Geometry: final body of the model. Coordinates: model frame, mm. Face numbers are marked on the shaded views. A direction names the side the tool comes from. Give positions to 0.01 mm unless a question says otherwise; leave off trailing zeros. Loops run counter-clockwise (first coordinate to the right, second up) from the corner with the lowest first, then second, coordinate; pieces in that order, holes last.
1. Section D-D, the plane x = 13.5. Output: boundary loops of the cut face in (y, z) (3 decimals), then the cut area to 3 significant figures.
2. First-contact query: P1, Ø8, axis at x = 0, y = -22.5, coming from the -Z side; P2, Ø1.6, axis at y = 2.5, z = 1, coming from the -X side; P3, Ø3, axis at x = -17, y = 14.5, coming from the +Z side; P4, Ø14, axis at x = -4.5, y = 25, coming from the +Z side (3 decimals). Flat tips, straight axial feed; report the tip coordinate or a pass-through.
3. Section C-C, the plane z = 43.5. Output: boundary loops of the cut face in (x, y), then the cut area to 3 significant figures.
4. Section B-B, the plane x = -10. Output: boundary loops of the cut face in (y, z) (3 decimals), then the cut area to 3 significant figures.
5. Material intervals for line 1 along Z through (x, y) = (-7.5, -28.5) (3 decimals); line 2 along Z through (x, y) = (-10, 11.5) (3 decimals); line 3 along X through (y, z) = (-14, 2.5), sorted ascending.
6. Access query for the marked faces 1, 2, 3 and 4. Directions: +Z, -Z, +X, -X, +Y, -Y. A direction counts if a zero-diameter tool reaches every point of the face in a straight line with its end or side. Return the directions, or none.
7. Section A-A, the plane y = -13.5. Output: boundary loops of the cut face in (x, z) (3 decimals), then the cut area to 3 significant figures.
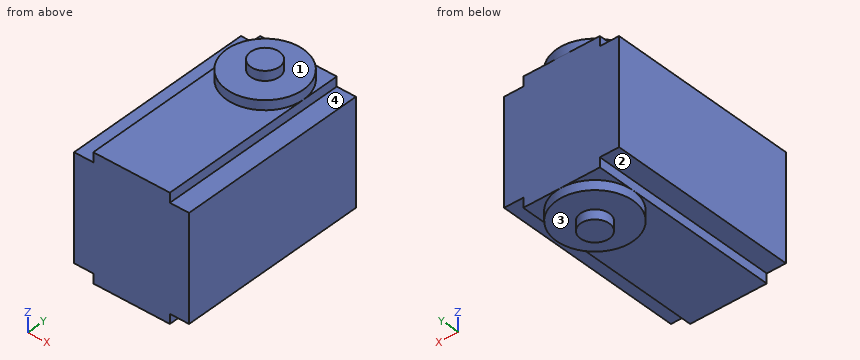
from build123d import *

# Parameters (mm, degrees)
SKETCH1_W           = 38.1
SKETCH1_H           = 63.5
BOSS_EXTRUDE1_DEPTH = 41.275
SKETCH2_R           = 12.7
BOSS_EXTRUDE2_DEPTH = 3.175
SKETCH3_R           = 4.7625
BOSS_EXTRUDE3_DEPTH = 3.175
SKETCH5_W           = 6.35
SKETCH5_H           = 63.5
CUT_EXTRUDE1_DEPTH  = 3.175


with BuildPart() as part:
    # Sketch1 → Boss-Extrude1 (new body)
    with BuildSketch(Plane.XY):
        Rectangle(SKETCH1_W, SKETCH1_H)
    extrude(amount=BOSS_EXTRUDE1_DEPTH)

    # Sketch2 → Boss-Extrude2 (add)
    with BuildSketch(Plane(origin=(0, 0, 0), x_dir=(-1, 0, 0), z_dir=(0, 0, -1))):
        with Locations((0, 19.05)):
            Circle(SKETCH2_R)
    boss_extrude2 = extrude(amount=BOSS_EXTRUDE2_DEPTH)

    # Sketch3 → Boss-Extrude3 (add)
    with BuildSketch(Plane(origin=(0, 0, -3.175), x_dir=(-1, 0, 0), z_dir=(0, 0, -1))):
        with Locations((0, 19.05)):
            Circle(SKETCH3_R)
    boss_extrude3 = extrude(amount=BOSS_EXTRUDE3_DEPTH)

    # Mirror1: Boss-Extrude2, Boss-Extrude3 across plane
    add(boss_extrude2.mirror(Plane(origin=(0, 0, 20.6375), x_dir=(1, 0, 0), z_dir=(0, 0, -1))))
    add(boss_extrude3.mirror(Plane(origin=(0, 0, 20.6375), x_dir=(1, 0, 0), z_dir=(0, 0, -1))))

    # Sketch5 → Cut-Extrude1 (cut)
    with BuildSketch(Plane.XY.offset(41.275)):
        with Locations((-15.875, 0)):
            Rectangle(SKETCH5_W, SKETCH5_H)
        with Locations((15.875, 0)):
            Rectangle(SKETCH5_W, SKETCH5_H)
    cut_extrude1 = extrude(amount=-CUT_EXTRUDE1_DEPTH, mode=Mode.SUBTRACT)

    # Mirror2: Cut-Extrude1 across plane
    add(cut_extrude1.mirror(Plane(origin=(0, 0, 20.6375), x_dir=(1, 0, 0), z_dir=(0, 0, -1))), mode=Mode.SUBTRACT)


solid = part.part
Answers below:
1. outline: (-31.75, 3.175) - (31.75, 3.175) - (31.75, 38.1) - (-31.75, 38.1) - close
1. area: 2,220 mm2
2. P1: stops at z = 0
2. P2: stops at x = -12.7
2. P3: stops at z = 38.1
2. P4: stops at z = 47.625
3. outline: circle Ø25.4 at (0, 19.05)
3. area: 507 mm2
4. outline: (-31.75, 0) - (11.221, 0) - (11.221, -3.175) - (26.879, -3.175) - (26.879, 0) - (31.75, 0) - (31.75, 41.275) - (26.879, 41.275) - (26.879, 44.45) - (11.221, 44.45) - (11.221, 41.275) - (-31.75, 41.275) - close
4. area: 2,720 mm2
5. line 1: z = 0 to 41.275
5. line 2: z = -3.175 to 44.45
5. line 3: x = -12.7 to 12.7
6. face 1: +Z
6. face 2: -Z, -X, +Y, -Y
6. face 3: -Z
6. face 4: +Z, +X, +Y, -Y
7. outline: (-19.05, 3.175) - (-12.7, 3.175) - (-12.7, 0) - (12.7, 0) - (12.7, 3.175) - (19.05, 3.175) - (19.05, 38.1) - (12.7, 38.1) - (12.7, 41.275) - (-12.7, 41.275) - (-12.7, 38.1) - (-19.05, 38.1) - close
7. area: 1,490 mm2
